from build123d import *

# Parameters (mm, degrees)
F0_W     = 406.4
F0_H     = 76.2
F1_DEPTH = 12.7
F3_DEPTH = 62.484
F5_DEPTH = 38.608


with BuildPart() as f1:
    # F0 (on Right) → F1 (new body)
    with BuildSketch(Plane.YZ):
        Rectangle(F0_W, F0_H)
    extrude(amount=F1_DEPTH)

    # F2 (on face) → F3 (cut)
    with BuildSketch(Plane.YZ.offset(12.7)):
        with BuildLine():
            Line((50.8, 25.4), (-50.8, 25.4))
            ThreePointArc((-50.8, 25.4), (-55.290128, 23.540128), (-57.15, 19.05))
            Line((-57.15, 19.05), (-57.15, -6.35))
            ThreePointArc((-57.15, -6.35), (-55.290128, -10.840128), (-50.8, -12.7))
            Line((-50.8, -12.7), (50.8, -12.7))
            ThreePointArc((50.8, -12.7), (55.290128, -10.840128), (57.15, -6.35))
            Line((57.15, -6.35), (57.15, 19.05))
            ThreePointArc((57.15, 19.05), (55.290128, 23.540128), (50.8, 25.4))
        make_face()
    extrude(amount=-F3_DEPTH, mode=Mode.SUBTRACT)

    # F4 (on face) → F5 (cut)
    with BuildSketch(Plane.YZ.offset(12.7)):
        with BuildLine():
            Line((-203.2, 38.1), (-203.2, 0))
            ThreePointArc((-203.2, 0), (-173.311901, 2.959505), (-144.584615, 11.723077))
            Line((-144.584615, 11.723077), (-109.415385, 26.376923))
            ThreePointArc((-109.415385, 26.376923), (-80.688099, 35.140495), (-50.8, 38.1))
            Line((-50.8, 38.1), (-203.2, 38.1))
        make_face()
        with BuildLine():
            Line((109.415385, 26.376923), (144.584615, 11.723077))
            ThreePointArc((144.584615, 11.723077), (173.311901, 2.959505), (203.2, 0))
            Line((203.2, 0), (203.2, 38.1))
            Line((203.2, 38.1), (50.8, 38.1))
            ThreePointArc((50.8, 38.1), (80.688099, 35.140495), (109.415385, 26.376923))
        make_face()
    extrude(amount=-F5_DEPTH, mode=Mode.SUBTRACT)


solid = f1.part
Could you check a few things on this model? Use its own coordinates, in mm. A direction names the side the tool comes from. Give positions to 0.01 mm unless a question says otherwise; leave off trailing zeros. Order: outer loops, then holes, each group sorted by start corner. A loop starts at its lowest first (then second) coordinate and runs counter-clockwise, first axis right, second up.
Item 1: I need wall thicknesses on line 1 (Z direction, x = 7, y = 48); line 2 (Y direction, x = 0.5, z = -7); line 3 (Y direction, x = 11, z = 20). Which ranges of each line are inside material? Lowest first, please.
Item 2: If we section it at D-D, the plane y = -173.5: Write out the boundary of the cut face in (x, z), plus the area to 3 significant figures.
Item 3: If we section it at A-A, the plane y = -2: Write out the boundary of the cut face in (x, z).
Item 4: For faces 4 (the face through (6.44, 55.24, -10.89)), 5 (the face through (0, -3, -16)), which set-ups out of +Z, -Z, +X, -X, +Y, -Y let a thin tool reach every point of the face, with its end or its side?
Item 5: If we section it at C-C, the plane y = 77: Write out the boundary of the cut face in (x, z), plus the area to 3 significant figures.
Item 6: If we mould it in two halves opening along Z, with no side actions, what happens to faces 1 (the face through (6.44, -55.24, 23.59)), 2 (the face through (6.44, -173.72, 2.88)), 3 (the face through (6, -3, -38.1))? For each: pulls with the +Z half, pulls with the -Z half, needs draft (parallel to the pull), parting line crosses it, or undercut.
Item 7: I'm going to push flat-ended pins straight in: pin 1 (5 mm diameter, centred on x = 7.5, z = 23, fed in from -Y); pin 2 (1.5 mm diameter, centred on x = 10.5, y = -142.5, fed in from +Z). Where does each tip first touch, or does it pass through?
Item 8: If we section it at B-B, the plane x = 4: Write out the boundary of the cut face in (y, z).
Values:
1. line 1: z = -38.1 to -12.7, 25.4 to 38.1
1. line 2: y = -203.2 to -57.12, 57.12 to 203.2
1. line 3: y = -124.72 to -57.08, 57.08 to 124.72
2. outline: (0, -38.1) - (12.7, -38.1) - (12.7, 2.92) - (0, 2.92) - close
2. area: 521 mm2
3. outline: (0, -38.1) - (12.7, -38.1) - (12.7, -12.7) - (0, -12.7) - close; (0, 25.4) - (12.7, 25.4) - (12.7, 38.1) - (0, 38.1) - close
4. face 4: +X, -X
4. face 5: +Z, -Z, -X, +Y, -Y
5. outline: (0, -38.1) - (12.7, -38.1) - (12.7, 35.83) - (0, 35.83) - close
5. area: 939 mm2
6. face 1: undercut
6. face 2: pulls with the +Z half
6. face 3: pulls with the -Z half
7. pin 1: stops at y = -123.52
7. pin 2: stops at z = 12.9
8. outline: (-203.2, -38.1) - (203.2, -38.1) - (203.2, 0) arc R152.4 cw to (144.58, 11.72) - (109.42, 26.38) arc R152.4 ccw to (50.8, 38.1) - (-50.8, 38.1) arc R152.4 ccw to (-109.42, 26.38) - (-144.58, 11.72) arc R152.4 cw to (-203.2, 0) - close; hole (-57.15, -6.35) arc R6.35 ccw to (-50.8, -12.7) - (50.8, -12.7) arc R6.35 ccw to (57.15, -6.35) - (57.15, 19.05) arc R6.35 ccw to (50.8, 25.4) - (-50.8, 25.4) arc R6.35 ccw to (-57.15, 19.05) - close
